Geometry check sheet. Reference: the model listing, model coordinates, mm. Round coordinates to 2 decimals unless told otherwise and drop trailing zeros. Write each loop counter-clockwise with the first axis right and the second up, starting at its lowest first coordinate (ties: lowest second). Pieces come first, ordered by that corner, then holes.
Item 1: Depth check by flat-ended pin: P1, Ø1.5, axis at x = 0, y = 0, coming from the -Z side. Enter the tip coordinate at first touch or a pass-through.
Item 2: Cross-section at C-C (y = 9.5). Enter the section's corners in (x, z).
Item 3: Cross-section at A-A (x = 0). Enter the section's corners in (y, z), then the cut area to 3 significant figures.
Item 4: Draft check along X on faces 1 (the face through (-7, 7, 5.08)), 2 (the face through (-0.936, 0.858, 2.12)), 3 (the face through (-12.7, 0, 3)), 4 (the face through (-0.03, 6.72, 3.81)). Enter one of: pulls with the +X half, pulls with the -X half, needs draft (parallel to the pull), parting line crosses it, or undercut.
Item 5: Scan lines: probe 1 along Y at (x, z) = (0, 3.4); probe 2 along Z at (x, y) = (0, -9.5). Record each from-to range of solid material in increasing order.
from build123d import *

# Parameters (mm, degrees)
F0_W     = 25.4
F0_H     = 25.4
F1_DEPTH = 5.08
F3_DEPTH = 25.4
F5_DEPTH = 25.4
F6_R     = 1.27
F7_DEPTH = 25.4


with BuildPart() as f1:
    # F0 (on Top) → F1 (new body)
    with BuildSketch(Plane.XY):
        Rectangle(F0_W, F0_H)
    extrude(amount=F1_DEPTH)

    # F2 (on face) → F3 (cut)
    with BuildSketch(Plane.YZ.offset(12.7)):
        with BuildLine():
            ThreePointArc((-1.27, 5.08), (0, 3.81), (1.27, 5.08))
            Line((1.27, 5.08), (-1.27, 5.08))
        make_face()
    extrude(amount=-F3_DEPTH, mode=Mode.SUBTRACT)

    # F4 (on face) → F5 (cut)
    with BuildSketch(Plane.XZ.offset(12.7)):
        with BuildLine():
            ThreePointArc((-1.27, 5.08), (0, 3.81), (1.27, 5.08))
            Line((1.27, 5.08), (-1.27, 5.08))
        make_face()
    extrude(amount=-F5_DEPTH, mode=Mode.SUBTRACT)

    # F6 (on face) → F7 (cut)
    with BuildSketch(Plane.XY.offset(5.08)):
        Circle(F6_R)
    extrude(amount=-F7_DEPTH, mode=Mode.SUBTRACT)


solid = f1.part
Resolved:
1. P1: passes through
2. outline: (-12.7, 0) - (12.7, 0) - (12.7, 5.08) - (1.27, 5.08) arc R1.27 cw to (-1.27, 5.08) - (-12.7, 5.08) - close
3. outline: (-12.7, 0) - (-1.27, 0) - (-1.27, 3.81) - (-12.7, 3.81) - close; (1.27, 0) - (12.7, 0) - (12.7, 3.81) - (1.27, 3.81) - close
3. area: 87.1 mm2
4. face 1: needs draft
4. face 2: undercut
4. face 3: pulls with the -X half
4. face 4: undercut
5. probe 1: y = -12.7 to -1.27, 1.27 to 12.7
5. probe 2: z = 0 to 3.81
